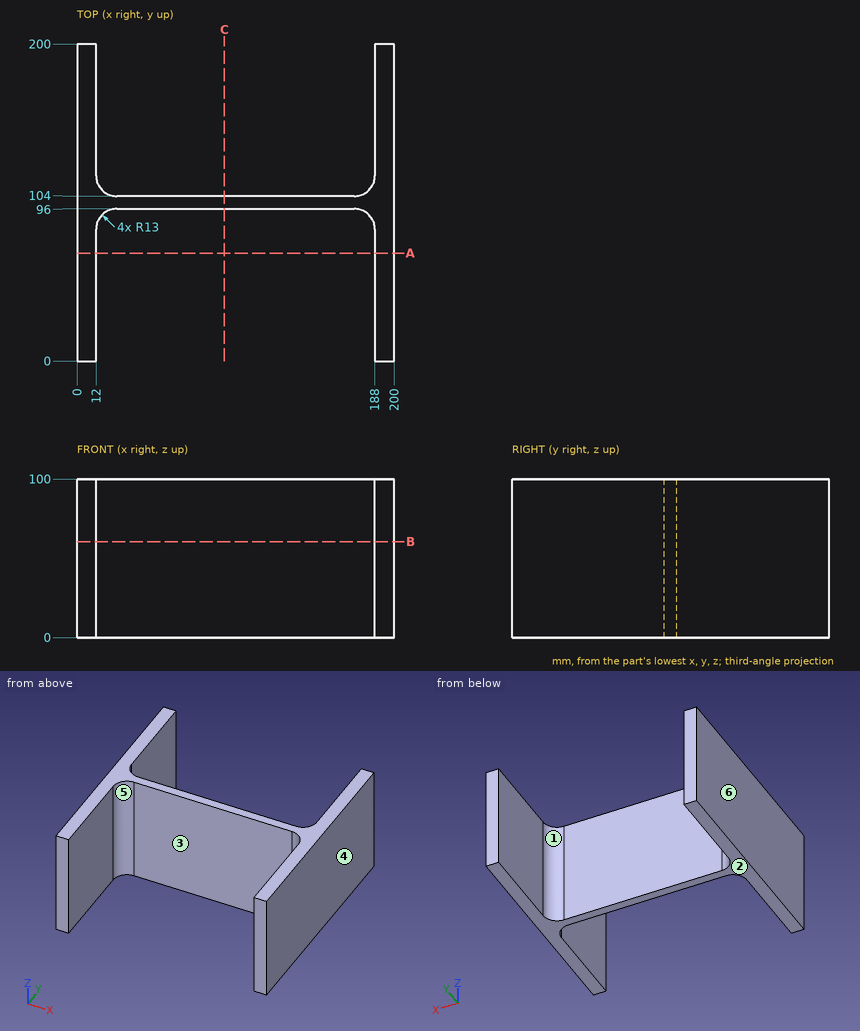
Drawing for the job (mm, zero at the part's lowest x, y, z). A direction names the side the tool comes from. Round coordinates to 2 decimals unless told otherwise and drop trailing zeros. Write each loop counter-clockwise with the first axis right and the second up, starting at its lowest first coordinate (ties: lowest second). Pieces come first, ordered by that corner, then holes. Notation, with made-up numbers: M 49,-26.5 L 82,-26.5 A12 cw 82,-21.5 Z; hole C 10,87.5 d3. An arc over 180 degrees is marked long. Answer in a Markdown table with one row per item.
1. Saw through at B-B (z = 60.5). List the corners of the cut face in (x, y).
Geometry check:
| item | result |
|---|---|
| outline | M 0,0 L 12,0 L 12,83 A13 cw 25,96 L 175,96 A13 cw 188,83 L 188,0 L 200,0 L 200,200 L 188,200 L 188,117 A13 cw 175,104 L 25,104 A13 cw 12,117 L 12,200 L 0,200 Z |
2. Mould opens along X. For the marked faces 4, 5 and 6 say: +X half, -X half, draft (parallel to the pull), parting line (faces both ways), or undercut.
Geometry check:
| item | result |
|---|---|
| face 4 | +X half |
| face 5 | undercut |
| face 6 | -X half |
3. Flat gauge pins, fed straight in: P1, Ø6, axis at x = 55, z = 62.5, coming from the +Y side; P2, Ø1, axis at x = 107, y = 105.5, coming from the +Z side. Where does each tip first touch, or does it go through?
Geometry check:
| item | result |
|---|---|
| P1 | y = 104 |
| P2 | through |
4. Probe L1, parallel to X at y = 161, z = 25; L2, parallel to Y at x = 103, z = 82.5; L3, parallel to X at y = 109, z = 94. List the from-to ranges inside material, lowest first. Write a range as [from, to].
Geometry check:
| item | result |
|---|---|
| L1 | [0, 12], [188, 200] |
| L2 | [96, 104] |
| L3 | [0, 14.75], [185.25, 200] |
5. Saw through at A-A (y = 68). List the corners of the cut face in (x, z), and give its area (3 significant figures).
Geometry check:
| item | result |
|---|---|
| outline | M 0,0 L 12,0 L 12,100 L 0,100 Z; M 188,0 L 200,0 L 200,100 L 188,100 Z |
| area | 2,400 mm2 |
6. Saw through at C-C (x = 93). List the corners of the cut face in (y, z), and give its area (3 significant figures).
Geometry check:
| item | result |
|---|---|
| outline | M 96,0 L 104,0 L 104,100 L 96,100 Z |
| area | 800 mm2 |
7. Which spindle directions (+Z, -Z, +X, -X, +Y, -Y) get a long thin tool onto all of the face, cutting with end or side? Do the marked faces 1, 2 and 3. Say none if no direction does.
Geometry check:
| item | result |
|---|---|
| face 1 | +Z, -Z, +Y |
| face 2 | -Z, +X, -X, +Y, -Y |
| face 3 | +Z, -Z, -Y |
